```python
from build123d import *

# Parameters (mm, degrees)
SKETCH013_R     = 3.5
SKETCH013_R_2   = 1.6
SKETCH013_W     = 7
SKETCH013_H     = 7
PAD004_DEPTH    = 3.5
PAD_DEPTH       = 10
SKETCH015_R     = 1.15
POCKET005_DEPTH = 5
SKETCH004_R     = 1
POCKET006_DEPTH = 5
SKETCH014_R     = 1.75
POCKET007_DEPTH = 5
POCKET_DEPTH    = 2


with BuildPart() as part:
    # Sketch013 → Pad004 (new body)
    with BuildSketch(Plane.XY):
        Polygon((0, 65), (150, 65.000002), (150, -65), (0, -65), align=None)
        with Locations((13, 25)):
            Circle(SKETCH013_R, mode=Mode.SUBTRACT)
        with Locations((58, 25)):
            Circle(SKETCH013_R, mode=Mode.SUBTRACT)
        with Locations((13, -30)):
            Circle(SKETCH013_R, mode=Mode.SUBTRACT)
        with Locations((58, -30)):
            Circle(SKETCH013_R, mode=Mode.SUBTRACT)
        with Locations((146, 61.000002)):
            Circle(SKETCH013_R_2, mode=Mode.SUBTRACT)
        with Locations((146, -61)):
            Circle(SKETCH013_R_2, mode=Mode.SUBTRACT)
        with Locations((81.000022, 44.539576)):
            Circle(SKETCH013_R_2, mode=Mode.SUBTRACT)
        with Locations((136, 44.539576)):
            Circle(SKETCH013_R_2, mode=Mode.SUBTRACT)
        with Locations((80.901087, -45.46037)):
            Circle(SKETCH013_R_2, mode=Mode.SUBTRACT)
        with Locations((135.901066, -45.46037)):
            Circle(SKETCH013_R_2, mode=Mode.SUBTRACT)
        with Locations((90.500022, 44.539576)):
            Rectangle(SKETCH013_W, SKETCH013_H, mode=Mode.SUBTRACT)
        with Locations((108.500011, 44.519789)):
            Rectangle(SKETCH013_W, SKETCH013_H, mode=Mode.SUBTRACT)
        with Locations((126.5, 44.500002)):
            Rectangle(SKETCH013_W, SKETCH013_H, mode=Mode.SUBTRACT)
        with Locations((90.480235, 26.539587)):
            Rectangle(SKETCH013_W, SKETCH013_H, mode=Mode.SUBTRACT)
        with Locations((108.480224, 26.5198)):
            Rectangle(SKETCH013_W, SKETCH013_H, mode=Mode.SUBTRACT)
        with Locations((126.480213, 26.500013)):
            Rectangle(SKETCH013_W, SKETCH013_H, mode=Mode.SUBTRACT)
        with Locations((90.460448, 8.539598)):
            Rectangle(SKETCH013_W, SKETCH013_H, mode=Mode.SUBTRACT)
        with Locations((108.460437, 8.519811)):
            Rectangle(SKETCH013_W, SKETCH013_H, mode=Mode.SUBTRACT)
        with Locations((126.460426, 8.500024)):
            Rectangle(SKETCH013_W, SKETCH013_H, mode=Mode.SUBTRACT)
        with Locations((90.440661, -9.460392)):
            Rectangle(SKETCH013_W, SKETCH013_H, mode=Mode.SUBTRACT)
        with Locations((108.44065, -9.480178)):
            Rectangle(SKETCH013_W, SKETCH013_H, mode=Mode.SUBTRACT)
        with Locations((126.440639, -9.499965)):
            Rectangle(SKETCH013_W, SKETCH013_H, mode=Mode.SUBTRACT)
        with Locations((90.420874, -27.460381)):
            Rectangle(SKETCH013_W, SKETCH013_H, mode=Mode.SUBTRACT)
        with Locations((108.420863, -27.480168)):
            Rectangle(SKETCH013_W, SKETCH013_H, mode=Mode.SUBTRACT)
        with Locations((126.420852, -27.499954)):
            Rectangle(SKETCH013_W, SKETCH013_H, mode=Mode.SUBTRACT)
        with Locations((90.401087, -45.46037)):
            Rectangle(SKETCH013_W, SKETCH013_H, mode=Mode.SUBTRACT)
        with Locations((108.401076, -45.480157)):
            Rectangle(SKETCH013_W, SKETCH013_H, mode=Mode.SUBTRACT)
        with Locations((126.401066, -45.499944)):
            Rectangle(SKETCH013_W, SKETCH013_H, mode=Mode.SUBTRACT)
    extrude(amount=PAD004_DEPTH)

    # Sketch001 → Pad (join)
    with BuildSketch(Plane.XY.offset(3.5)):
        Polygon((0, 55), (3, 55), (128, 55), (128, 50), (3, 50), (3, -60), (128, -60), (128, -65), (3, -65), (0, -65), align=None)
    extrude(amount=PAD_DEPTH)

    # Sketch015 → Pocket005 (cut)
    with BuildSketch(Plane.XZ.offset(65)):
        with Locations((53, 7)):
            Circle(SKETCH015_R)
    extrude(amount=-POCKET005_DEPTH, mode=Mode.SUBTRACT)

    # Sketch004 → Pocket006 (cut, symmetric)
    with BuildSketch(Plane.XZ.offset(-55)):
        with Locations((25, 9)):
            Circle(SKETCH004_R)
        with Locations((95, 9)):
            Circle(SKETCH004_R)
        with Locations((55, 9)):
            Circle(SKETCH004_R)
        with Locations((125, 9)):
            Circle(SKETCH004_R)
    extrude(amount=POCKET006_DEPTH, both=True, mode=Mode.SUBTRACT)

    # Sketch014 → Pocket007 (cut)
    with BuildSketch(Plane.YZ):
        with Locations((45, 8)):
            Circle(SKETCH014_R)
        with Locations((-5, 8)):
            Circle(SKETCH014_R)
        with Locations((-55, 8)):
            Circle(SKETCH014_R)
    extrude(amount=POCKET007_DEPTH, mode=Mode.SUBTRACT)

    # Sketch → Pocket (cut)
    with BuildSketch(Plane.XY.offset(3.5)):
        Polygon((83.55, 52), (134.15, 52), (134.15, 42.5), (140, 42.5), (140, -42.5), (134.15, -42.5), (134.15, -53), (83.55, -53), (83.55, -42.5), (72.55, -42.5), (72.55, 42.5), (83.55, 42.5), align=None)
    extrude(amount=-POCKET_DEPTH, mode=Mode.SUBTRACT)


solid = part.part
```
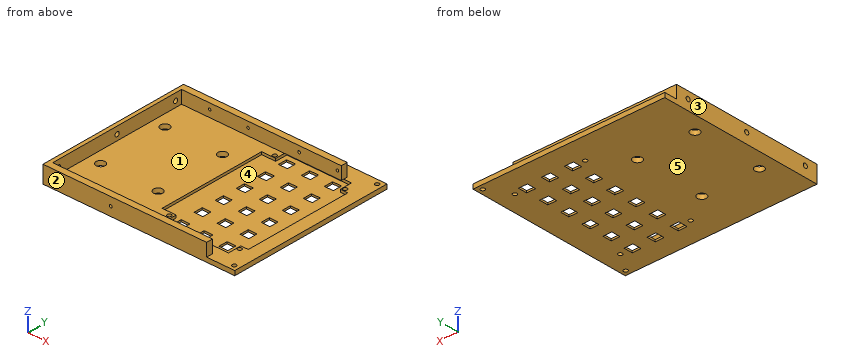
Read the model definition and answer for the solid it produces. Units are mm, in the model's axes. Face numbers are marked on the shaded views. A direction names the side the tool comes from. Coordinates: 2 decimals unless noted, no trailing zeros. Loops run counter-clockwise (first coordinate to the right, second up) from the corner with the lowest first, then second, coordinate; pieces in that order, holes last.
(1) A tool of negligible diameter and unlimited length cuts with its end or side. For the marked faces 1 and 2, from which of +Z, -Z, +X, -X, +Y, -Y can it reach the whole face along a straight path? Write none if from no direction.
Solution:
face 1: +Z, +X
face 2: +Z, -Z, +X, -X, -Y
(2) Consider line 1 along X through (y, z) = (46.5, 0.5); line 2 along Y through (x, z) = (132, 2); line 3 along Y through (x, z) = (64, 7). Determine where each line is inside the solid, lowest interval first.
Solution:
line 1: x = 0 to 87, 94 to 105, 112 to 123, 130 to 150
line 2: y = -65 to -53, 52 to 65
line 3: y = -65 to -60, 50 to 55
(3) The mould has two halves that part along X. Classify the marked faces 3, 4 and 5: released by +X, released by -X, zero draft, split by the parting line, or undercut.
Solution:
face 3: released by -X
face 4: undercut
face 5: zero draft
(4) The part is cut by section C-C (y = -55). Determine the outline of the cut face in (x, z), and give its area (4 significant figures).
Solution:
outline: (0, 0) - (150, 0) - (150, 3.5) - (3, 3.5) - (3, 6.25) - (0, 6.25) - close; (0, 9.75) - (3, 9.75) - (3, 13.5) - (0, 13.5) - close
area: 544.5 mm2
(5) The part is cut by section D-D (x = 46.5). Determine the outline of the cut face in (y, z), and give its area (3 significant figures).
Solution:
outline: (-65, 0) - (65, 0) - (65, 3.5) - (55, 3.5) - (55, 13.5) - (50, 13.5) - (50, 3.5) - (-60, 3.5) - (-60, 13.5) - (-65, 13.5) - close
area: 555 mm2
(6) Flat-ended cylindrical pins translate along their axes: pin 1 Ø4 at (x, y) = (121, 46) entering from +Z; pin 2 Ø5 at (x, z) = (30.5, 11) entering from +Y; pin 3 Ø3 at (y, z) = (20, 6) entering from +X. Find the tip coordinate at first contact, or state that the pin passes through.
Solution:
pin 1: stops at z = 1.5
pin 2: stops at y = 55
pin 3: stops at x = 3
(7) The part is cut by section B-B (y = 25). Count the separate pieces of the cut face and the enclosed holes in it, and give its area (3 significant figures).
Solution:
separate pieces: 6
enclosed holes: 0
area: 340 mm2
(8) The part is cut by section A-A (x = 13). Determine the outline of the cut face in (y, z).
Solution:
outline: (-65, 0) - (-33.5, 0) - (-33.5, 3.5) - (-60, 3.5) - (-60, 13.5) - (-65, 13.5) - close; (-26.5, 0) - (21.5, 0) - (21.5, 3.5) - (-26.5, 3.5) - close; (28.5, 0) - (65, 0) - (65, 3.5) - (55, 3.5) - (55, 13.5) - (50, 13.5) - (50, 3.5) - (28.5, 3.5) - close
